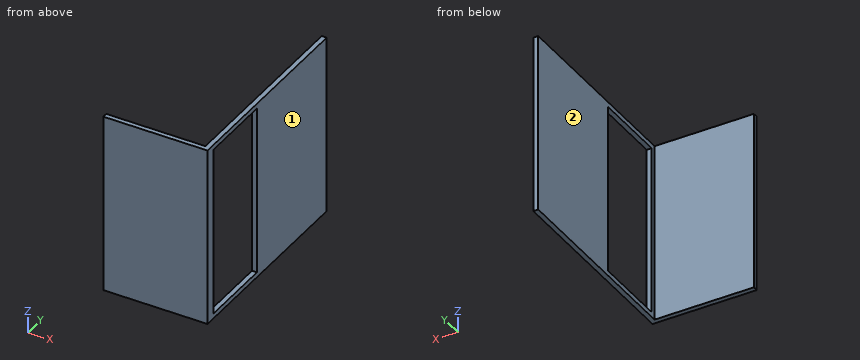
Autodesk Inventor part; units mm, degrees
ref_plane "YZ Plane" through (0, 0, 0) normal (1, 0, 0) x (0, 1, 0)
ref_plane "XZ Plane" through (0, 0, 0) normal (0, 1, 0) x (-1, 0, 0)
ref_plane "XY Plane" through (0, 0, 0) normal (0, 0, 1) x (1, 0, 0)
sketch "Sketch1" plane through (0, 0, 0) normal (0, 1, 0) x (-1, 0, 0)
  line L0 (0, 0) -> (106.68, 0)
  line L1 (106.68, 0) -> (106.68, -184.15)
  line L2 (106.68, -184.15) -> (0, -184.15)
  line L3 (0, -184.15) -> (0, 0)
  dimension "d0" = 184.15
  dimension "d1" = 106.68
extrude "Extrusion1" add sketch "Sketch1" along normal blind 5.08
sketch "Sketch2" plane through (0, 5.08, 0) normal (0, 1, 0) x (1, 0, 0)
  line L0 (-5.08, 0) -> (-5.08, 184.15)
  line L1 (0, 0) -> (0, 184.15)
  line L2 (-5.08, 0) -> (0, 0)
  line L3 (0, 184.15) -> (-106.68, 184.15)
  line L4 (-5.08, 184.15) -> (0, 184.15)
  dimension "d4" = 5.08
extrude "Extrusion2" add sketch "Sketch2" along normal blind 203.2
sketch "Sketch3" plane through (-5.08, 5.08, -184.15) normal (-1, 0, 0) x (0, 0, 1)
  line L0 (179.07, 5.08) -> (5.08, 5.08)
  line L1 (5.08, 5.08) -> (5.08, 81.28)
  line L2 (5.08, 81.28) -> (179.07, 81.28)
  line L3 (179.07, 81.28) -> (179.07, 5.08)
  line L4 (184.15, 0) -> (184.15, 203.2)
  line L5 (0, 0) -> (0, 203.2)
  line L6 (0, -5.08) -> (184.15, -5.08)
  dimension "d7" = 5.08
  dimension "d8" = 5.08
  dimension "d9" = 10.16
  dimension "d10" = 76.2
extrude "Extrusion3" cut sketch "Sketch3" against normal up to surface (5.08 mm away)
properties part number "Box_Bottom"
Part model, mm, in its own coordinate system. Face numbers are marked on the shaded views. A direction names the side the tool comes from. Give positions to 0.01 mm unless a question says otherwise; leave off trailing zeros. Order: outer loops, then holes, each group sorted by start corner. A loop starts at its lowest first (then second) coordinate and runs counter-clockwise, first axis right, second up. Notation, with made-up numbers: (16.25, -26.5) - (22.25, -26.5) arc R21 cw to (22.25, -17.5) - close; hole circle Ø6 at (82, 26.5). An arc over 180 degrees is marked (long way). Use one line per item in the form item = value.
Item 1: Probe probe 1 along Y at (x, z) = (-5, -145.5); probe 2 along X at (y, z) = (96, -152); probe 3 along Y at (x, z) = (-27, -89.5). List the from-to ranges inside material, lowest first. Write a range as from..to.
Solution:
probe_1 = 0..10.16, 86.36..208.28
probe_2 = -5.08..0
probe_3 = 0..5.08
Item 2: Which spindle directions (+Z, -Z, +X, -X, +Y, -Y) get a long thin tool onto all of the face, cutting with end or side? Do the marked faces 1 and 2. Say none if no direction does.
Solution:
face_1 = +Z, -Z, +X, +Y, -Y
face_2 = +Z, -Z, -X, +Y
Item 3: Slice it at C-C on x = -40. Give the cut face in (y, z), and give its area (3 significant figures).
Solution:
outline = (0, -184.15) - (5.08, -184.15) - (5.08, 0) - (0, 0) - close
area = 935 mm2
Item 4: Slice it at A-A on y = 41.5. Give the cut face in (x, z), and give its area (3 significant figures).
Solution:
outline = (-5.08, -184.15) - (0, -184.15) - (0, -179.07) - (-5.08, -179.07) - close; (-5.08, -5.08) - (0, -5.08) - (0, 0) - (-5.08, 0) - close
area = 51.6 mm2
Item 5: Pin check, flat tip, straight feed: pin 1 Ø1.5 at (x, z) = (-89, -136.5) entering from +Y. Stop position of the tip, or through.
Solution:
pin_1 = 5.08
Item 6: Slice it at D-D on y = 165. Give the cut face in (x, z), and give its area (3 significant figures).
Solution:
outline = (-5.08, -184.15) - (0, -184.15) - (0, 0) - (-5.08, 0) - close
area = 935 mm2
Item 7: Slice it at B-B on z = -156. Give the cut face in (x, y), and give its area (3 significant figures).
Solution:
outline = (-106.68, 0) - (0, 0) - (0, 10.16) - (-5.08, 10.16) - (-5.08, 5.08) - (-106.68, 5.08) - close; (-5.08, 86.36) - (0, 86.36) - (0, 208.28) - (-5.08, 208.28) - close
area = 1,190 mm2
